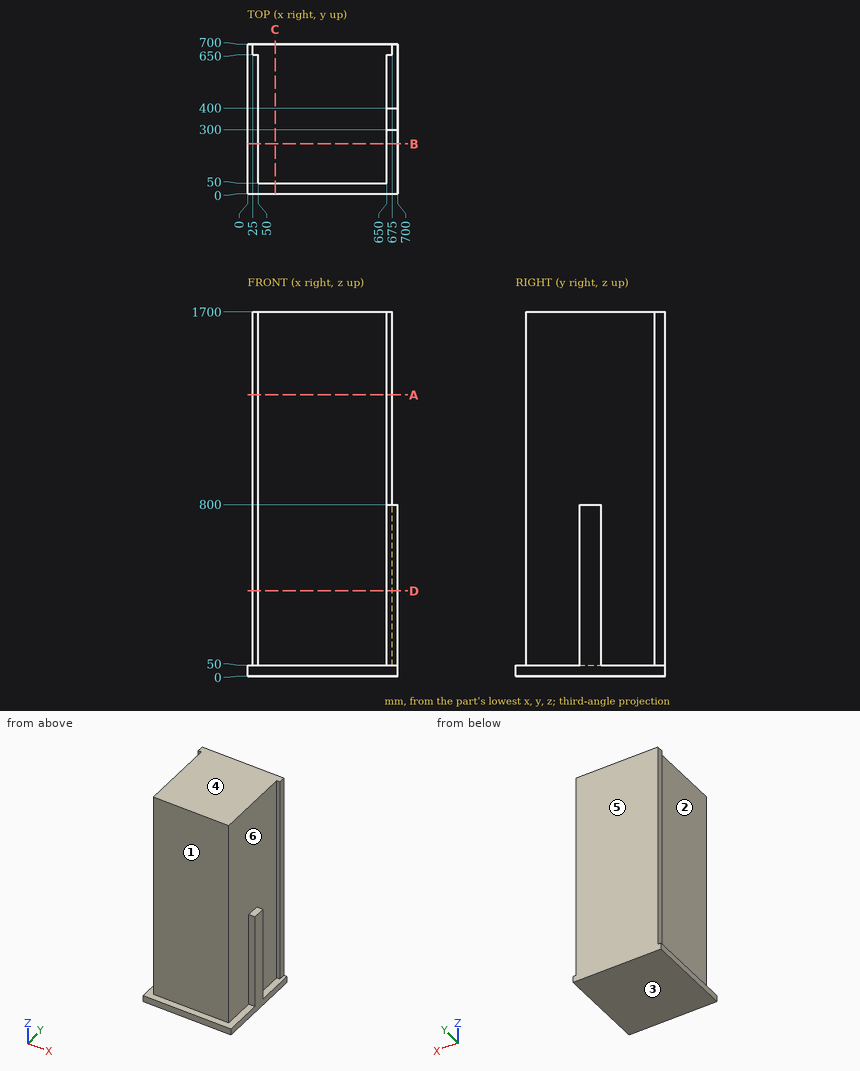
Study the drawing (mm; zero at the part's minimum x, y, z) and answer. A direction names the side the tool comes from. Give positions to 0.01 mm unless a question says otherwise; leave off trailing zeros. Order: outer loops, then holes, each group sorted by start corner. A loop starts at its lowest first (then second) coordinate and runs counter-clockwise, first axis right, second up. Notation, with made-up numbers: (55.5, -28) -> (108.5, -28) arc R28 ccw to (108.5, 5) -> close; hole circle Ø3 at (14, 57.25). An arc over 180 degrees is marked (long way). Write item = value, one per line.
1. Straight lines are drawn through the part: line 1 along X through (y, z) = (437, 264.5); line 2 along Y through (x, z) = (87.5, 1538); line 3 along X through (y, z) = (654.5, 1333). For each, find the intervals that lie inside material, in ascending order.
Numbers:
line_1 = 50 to 650
line_2 = 50 to 700
line_3 = 25 to 675
2. The mould has two halves that part along Y. Classify the marked faces 4, 5 and 6: +Y half, -Y half, draft (parallel to the pull), parting line (faces both ways), or undercut.
Numbers:
face_4 = draft
face_5 = +Y half
face_6 = undercut
3. A cutting plane is placed at C-C, the plane x = 129. Write down the section's boundary in (y, z), and give its area (3 significant figures).
Numbers:
outline = (0, 0) -> (700, 0) -> (700, 1700) -> (50, 1700) -> (50, 50) -> (0, 50) -> close
area = 1,110,000 mm²
4. Given pin 1 (3 mm diameter, centred on x = 575.5, z = 618.5, fed in from -Y); pin 2 (1.5 mm diameter, centred on y = 466, z = 1260, fed in from +X); pin 3 (8 mm diameter, centred on y = 173, z = 175, fed in from -X), each flat-ended and moving along its own axis, determine where each tip first touches the part or whether it passes through.
Numbers:
pin_1 = 50
pin_2 = 650
pin_3 = 50
5. For the marked faces 1, 2 and 3, determine the directions among +Z, -Z, +X, -X, +Y, -Y from which every point of the face is accessible in a straight line to the end or side of a thin tool.
Numbers:
face_1 = +Z, +X, -X, -Y
face_2 = +Z, -X, -Y
face_3 = -Z, +X, -X, +Y, -Y
6. A cutting plane is placed at A-A, the plane z = 1313. Write down the section's boundary in (x, y).
Numbers:
outline = (25, 650) -> (50, 650) -> (50, 50) -> (650, 50) -> (650, 650) -> (675, 650) -> (675, 700) -> (25, 700) -> close
7. A cutting plane is placed at D-D, the plane z = 397. Write down the section's boundary in (x, y), and give its area (4 significant figures).
Numbers:
outline = (25, 650) -> (50, 650) -> (50, 50) -> (650, 50) -> (650, 300) -> (700, 300) -> (700, 400) -> (650, 400) -> (650, 650) -> (675, 650) -> (675, 700) -> (25, 700) -> close
area = 397,500 mm²
8. A cutting plane is placed at B-B, the plane y = 233.5. Write down the section's boundary in (x, z), and give its area (4 significant figures).
Numbers:
outline = (0, 0) -> (700, 0) -> (700, 50) -> (650, 50) -> (650, 1700) -> (50, 1700) -> (50, 50) -> (0, 50) -> close
area = 1,025,000 mm²
